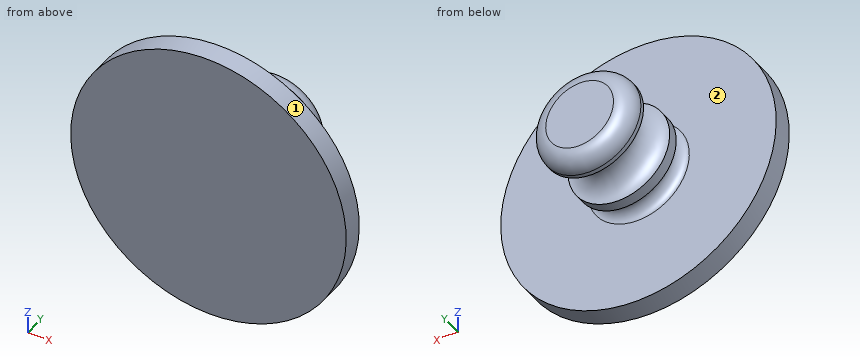
```python
from build123d import *


with BuildPart() as part:
    # Sketch1 → Revolve1 (revolve)
    with BuildSketch(Plane.XY, mode=Mode.PRIVATE) as revolve1_sk:
        with BuildLine():
            Line((0, 1), (0, 0))
            Line((0, 0), (6.5, 0))
            Line((6.5, 0), (6.5, 1))
            Line((6.5, 1), (2.4, 1))
            ThreePointArc((2.4, 1), (1.9, 1.5), (2.4, 2))
            Line((2.4, 2), (2.4, 2.5))
            ThreePointArc((2.4, 2.5), (1.4, 3.5), (2.4, 4.5))
            Line((2.4, 4.5), (2.4, 4.7))
            ThreePointArc((2.4, 4.7), (2.165685425, 5.265685425), (1.6, 5.5))
            Line((1.6, 5.5), (0, 5.5))
            Line((0, 5.5), (0, 1))
        make_face()
    revolve(revolve1_sk.sketch.rotate(Axis((0, 0, 0), (0, 1, 0)), 90), axis=Axis((0, 0, 0), (0, 1, 0)))


solid = part.part
```
Could you check a few things on this model? Use its own coordinates, in mm. Face numbers are marked on the shaded views. A direction names the side the tool comes from. Coordinates: 2 decimals unless noted, no trailing zeros. Loops run counter-clockwise (first coordinate to the right, second up) from the corner with the lowest first, then second, coordinate; pieces in that order, holes last.
1) Please list where these lines run through material, in increasing order: line 1 along Y through (x, z) = (5, -3); line 2 along Y through (x, z) = (1.5, -1); line 3 along X through (y, z) = (0.45, 3.75).
Reported:
line 1: y = 0 to 1
line 2: y = 0 to 2.7, 4.3 to 5.47
line 3: x = -5.31 to 5.31
2) Imagine slicing it at D-D (y = 3.7). List the corners of the cut face in (x, z) for me.
Reported:
outline: circle Ø2.84 at (0, 0)
3) Which directions (+Z, -Z, +X, -X, +Y, -Y) give clear straight access to the entire face, cutting with the end or side of a thin tool? Please do the marked faces 1 and 2.
Reported:
face 1: +Y, -Y
face 2: +Y
4) Imagine slicing it at B-B (x = 0). List the corners of the cut face in (y, z) for me, and give its area (3 significant figures).
Reported:
outline: (0, -6.5) - (1, -6.5) - (1, -2.4) arc R0.5 cw to (2, -2.4) - (2.5, -2.4) arc R1 cw to (4.5, -2.4) - (4.7, -2.4) arc R0.8 ccw to (5.5, -1.6) - (5.5, 1.6) arc R0.8 ccw to (4.7, 2.4) - (4.5, 2.4) arc R1 cw to (2.5, 2.4) - (2, 2.4) arc R0.5 cw to (1, 2.4) - (1, 6.5) - (0, 6.5) - close
area: 30.4 mm2
5) Will this pin go through, and if not, where does the flat tip stop? pin 1 Ø1 at (y, z) = (2.5, 2.5) entering from -X.
Reported:
pin 1: stops at x = -1.33
6) Imagine slicing it at C-C (y = 0.8). List the corners of the cut face in (x, z) for me, and give its area (3 significant figures).
Reported:
outline: circle Ø13 at (0, 0)
area: 133 mm2
7) Imagine slicing it at A-A (z = 0). List the corners of the cut face in (x, y) for me, and give its area (3 significant figures).
Reported:
outline: (-6.5, 0) - (6.5, 0) - (6.5, 1) - (2.4, 1) arc R0.5 cw to (2.4, 2) - (2.4, 2.5) arc R1 cw to (2.4, 4.5) - (2.4, 4.7) arc R0.8 ccw to (1.6, 5.5) - (-1.6, 5.5) arc R0.8 ccw to (-2.4, 4.7) - (-2.4, 4.5) arc R1 cw to (-2.4, 2.5) - (-2.4, 2) arc R0.5 cw to (-2.4, 1) - (-6.5, 1) - close
area: 30.4 mm2
